from build123d import *

# Parameters (mm, degrees)
SKETCH1_R           = 1.575
SKETCH1_R_2         = 1.5
BOSS_EXTRUDE1_DEPTH = 3
CUT_EXTRUDE1_DEPTH  = 45.467094576


with BuildPart() as part:
    # Sketch1 → Boss-Extrude1 (new, symmetric)
    with BuildSketch(Plane.XY):
        Polygon((-3.35, 6), (3.35, 6), (3.35, 3.05), (36.95, 3.05), (36.95, 6), (43.65, 6), (43.65, -6), (36.95, -6), (36.95, -3.05), (3.35, -3.05), (3.35, -6), (-3.35, -6), align=None)
        with Locations((40.3, 3)):
            Circle(SKETCH1_R, mode=Mode.SUBTRACT)
        with Locations((40.3, -3)):
            Circle(SKETCH1_R, mode=Mode.SUBTRACT)
        with Locations((0, 3)):
            Circle(SKETCH1_R_2, mode=Mode.SUBTRACT)
        with Locations((0, -3)):
            Circle(SKETCH1_R_2, mode=Mode.SUBTRACT)
    extrude(amount=BOSS_EXTRUDE1_DEPTH, both=True)

    # Sketch4 → Cut-Extrude1 (cut, through all)
    with BuildSketch(Plane.XY.offset(3)):
        with BuildLine():
            Line((10.273724121, 1), (30.026275879, 1))
            ThreePointArc((30.026275879, 1), (34.65, 0), (30.026275879, -1))
            Line((30.026275879, -1), (10.273724121, -1))
            ThreePointArc((10.273724121, -1), (5.65, 0), (10.273724121, 1))
        make_face()
    extrude(amount=-CUT_EXTRUDE1_DEPTH, mode=Mode.SUBTRACT)


solid = part.part
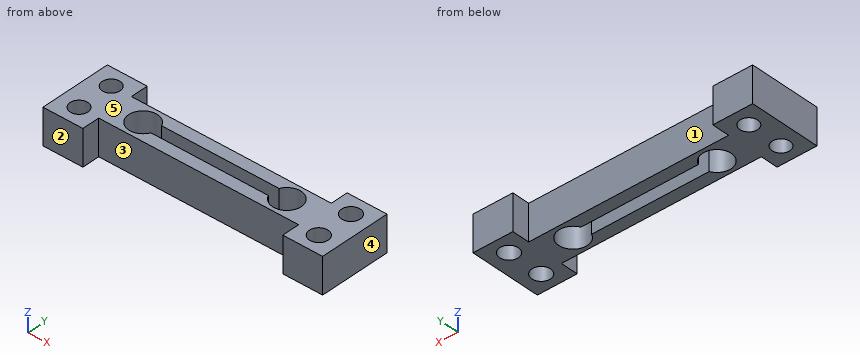
Build history of the part. All positions in model axes, mm. Face numbers are marked on the shaded views. A direction names the side the tool comes from. Give positions to 0.01 mm unless a question says otherwise; leave off trailing zeros. Loops run counter-clockwise (first coordinate to the right, second up) from the corner with the lowest first, then second, coordinate; pieces in that order, holes last. Notation, with made-up numbers: (65, -40) -> (100, -40) arc R4 cw to (100, -34) -> close; hole circle Ø4 at (-4.5, -37.75). An arc over 180 degrees is marked (long way). Answer in a Markdown table with one row per item.
Item 1: Slice it at D-D on y = 0. Write the cut outline in (x, z).
Findings below:
| item | result |
|---|---|
| outline | (-3.35, -3) -> (5.65, -3) -> (5.65, 3) -> (-3.35, 3) -> close; (34.65, -3) -> (43.65, -3) -> (43.65, 3) -> (34.65, 3) -> close |
Item 2: Slice it at C-C on z = -1.3. Write the cut outline in (x, y) (3 decimals).
Findings below:
| item | result |
|---|---|
| outline | (-3.35, -6) -> (3.35, -6) -> (3.35, -3.05) -> (36.95, -3.05) -> (36.95, -6) -> (43.65, -6) -> (43.65, 6) -> (36.95, 6) -> (36.95, 3.05) -> (3.35, 3.05) -> (3.35, 6) -> (-3.35, 6) -> close; hole circle Ø3 at (0, -3); hole circle Ø3 at (0, 3); hole (10.274, -1) -> (30.026, -1) arc R2.42 ccw (long way) to (30.026, 1) -> (10.274, 1) arc R2.42 ccw (long way) to start; hole circle Ø3.15 at (40.3, -3); hole circle Ø3.15 at (40.3, 3) |
Item 3: Tool access for the marked faces 1 and 2: list every direction of +Z, -Z, +X, -X, +Y, -Y with a clear straight run to the whole face (end or side of a thin tool).
Findings below:
| item | result |
|---|---|
| face 1 | +Z, -Z, +Y |
| face 2 | +Z, -Z, +X, -X, -Y |
Item 4: Flat gauge pins, fed straight in: P1, Ø1.8, axis at x = 23.5, z = -1, coming from the +Y side; P2, Ø3, axis at x = 18.5, z = -1, coming from the -Y side. Where does each tip first touch, or does it go through?
Findings below:
| item | result |
|---|---|
| P1 | stops at y = 3.05 |
| P2 | stops at y = -3.05 |
Item 5: Probe line 1 along Y through (x, z) = (0, 0.35); line 2 along Y through (x, z) = (29, -0.7); line 3 along X through (y, z) = (0, -1.5). List the from-to ranges inside material, lowest first. Write a range as [from, to].
Findings below:
| item | result |
|---|---|
| line 1 | y = [-6, -4.5], [-1.5, 1.5], [4.5, 6] |
| line 2 | y = [-3.05, -1], [1, 3.05] |
| line 3 | x = [-3.35, 5.65], [34.65, 43.65] |
Item 6: Mould opens along X. For the marked faces 3, 4 and 5 say: pulls with the +X half, pulls with the -X half, needs draft (parallel to the pull), parting line crosses it, or undercut.
Findings below:
| item | result |
|---|---|
| face 3 | undercut |
| face 4 | pulls with the +X half |
| face 5 | needs draft |
Item 7: Slice it at A-A on x = 8.07. Write the cut outline in (y, z).
Findings below:
| item | result |
|---|---|
| outline | (-3.05, -3) -> (-2.42, -3) -> (-2.42, 3) -> (-3.05, 3) -> close; (2.42, -3) -> (3.05, -3) -> (3.05, 3) -> (2.42, 3) -> close |
Item 8: Slice it at B-B on x = 40.3. Write the cut outline in (y, z) (3 decimals).
Findings below:
| item | result |
|---|---|
| outline | (-6, -3) -> (-4.575, -3) -> (-4.575, 3) -> (-6, 3) -> close; (-1.425, -3) -> (1.425, -3) -> (1.425, 3) -> (-1.425, 3) -> close; (4.575, -3) -> (6, -3) -> (6, 3) -> (4.575, 3) -> close |
